CAD build for the part. Positions are in the model's coordinates, mm. Coordinates: 2 decimals unless noted, no trailing zeros. Loops run counter-clockwise (first coordinate to the right, second up) from the corner with the lowest first, then second, coordinate; pieces in that order, holes last. Notation, with made-up numbers: (54, 16.25) -> (59, 16.25) arc R25 cw to (59, 36.25) -> close; hole circle Ø9 at (28, 35.5). An arc over 180 degrees is marked (long way). Write each question's results on one line, items separated by ' | '.
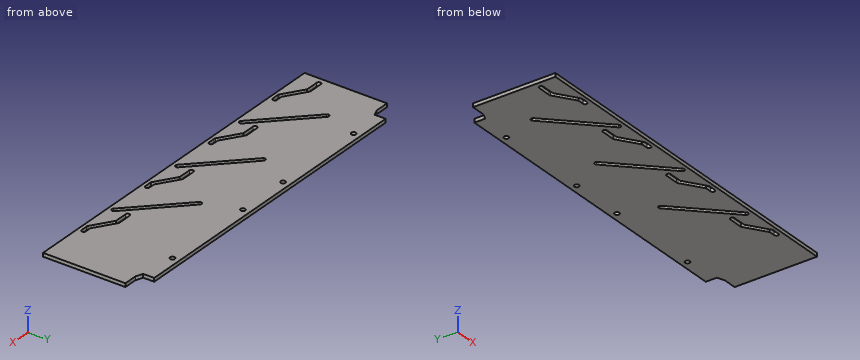
from build123d import *

# Parameters (mm, degrees)
SKETCH_1_W             = 260
SKETCH_1_H             = 70
EXTRUDE_1_DEPTH        = 2.6
SKETCH_2_R             = 1.7
CUT_EXTRUDE_1_DEPTH    = 135.654223848
SKETCH_3_R             = 1.3
CUT_EXTRUDE_2_DEPTH    = 135.654223848
CUT_EXTRUDE_4_DEPTH    = 135.654223848
PATTERN_LINEAR_2_COUNT = 3
PATTERN_LINEAR_2_PITCH = 63.333333333
CUT_EXTRUDE_3_DEPTH    = 135.654223848
PATTERN_LINEAR_1_COUNT = 4
PATTERN_LINEAR_1_PITCH = 63.333333333


with BuildPart() as part:
    # 草图1 → 凸台-拉伸1 (new body)
    with BuildSketch(Plane.XY):
        Rectangle(SKETCH_1_W, SKETCH_1_H)
    extrude(amount=EXTRUDE_1_DEPTH)

    # 草图2 → 切除-拉伸1 (cut, through all)
    with BuildSketch(Plane.XY.offset(2.6)):
        with Locations((-90, 30)):
            Circle(SKETCH_2_R)
        with Locations((-20, 30)):
            Circle(SKETCH_2_R)
        with Locations((20, 30)):
            Circle(SKETCH_2_R)
        with Locations((90, 30)):
            Circle(SKETCH_2_R)
        Polygon((-130, 25), (-130, 35), (-115, 35), (-115, 27), (-120, 25), align=None)
        Polygon((130, 25), (130, 35), (115, 35), (115, 27), (120, 25), align=None)
    extrude(amount=-CUT_EXTRUDE_1_DEPTH, mode=Mode.SUBTRACT)

    # 草图3 → 切除-拉伸2 (cut, through all)
    with BuildSketch(Plane.XY.offset(2.6)):
        with Locations((-61.666666667, -31)):
            Circle(SKETCH_3_R)
        with Locations((1.666666667, -31)):
            Circle(SKETCH_3_R)
        with Locations((65, -31)):
            Circle(SKETCH_3_R)
    extrude(amount=-CUT_EXTRUDE_2_DEPTH, mode=Mode.SUBTRACT)

    # 草图5 → 切除-拉伸4 (cut, through all)
    with BuildSketch(Plane.XY.offset(2.6)):
        with BuildLine():
            Line((-62.727326838, -32.060660172), (-98.727326838, 3.939339828))
            ThreePointArc((-98.727326838, 3.939339828), (-98.727326838, 6.060660172), (-96.606006495, 6.060660172))
            Line((-96.606006495, 6.060660172), (-60.606006495, -29.939339828))
            ThreePointArc((-60.606006495, -29.939339828), (-60.606006495, -32.060660172), (-62.727326838, -32.060660172))
        make_face()
    cut_extrude_4 = extrude(amount=-CUT_EXTRUDE_4_DEPTH, mode=Mode.SUBTRACT)

    # 阵列(线性)2: 切除-拉伸4 ×3
    with Locations(*[(i * PATTERN_LINEAR_2_PITCH, 0, 0) for i in range(1, PATTERN_LINEAR_2_COUNT)]):
        add(cut_extrude_4, mode=Mode.SUBTRACT)

    # 草图4 → 切除-拉伸3 (cut, through all)
    with BuildSketch(Plane.XY.offset(2.6)):
        with BuildLine():
            Line((-125, -19.5), (-115, -19.5))
            ThreePointArc((-115, -19.5), (-114.565323777, -19.56436196), (-114.167949706, -19.751924558))
            Line((-114.167949706, -19.751924558), (-99.545836543, -29.5))
            Line((-99.545836543, -29.5), (-95, -29.5))
            ThreePointArc((-95, -29.5), (-93.5, -31), (-95, -32.5))
            Line((-95, -32.5), (-100, -32.5))
            ThreePointArc((-100, -32.5), (-100.434676223, -32.43563804), (-100.832050294, -32.248075442))
            Line((-100.832050294, -32.248075442), (-115.454163457, -22.5))
            Line((-115.454163457, -22.5), (-125, -22.5))
            ThreePointArc((-125, -22.5), (-126.5, -21), (-125, -19.5))
        make_face()
    cut_extrude_3 = extrude(amount=-CUT_EXTRUDE_3_DEPTH, mode=Mode.SUBTRACT)

    # 阵列(线性)1: 切除-拉伸3 ×4
    with Locations(*[(i * PATTERN_LINEAR_1_PITCH, 0, 0) for i in range(1, PATTERN_LINEAR_1_COUNT)]):
        add(cut_extrude_3, mode=Mode.SUBTRACT)


solid = part.part
1) Slice it at C-C (y = -11). Write the cut outline in (x, z).
Outcome:
outline: (-130, 0) -> (-83.79, 0) -> (-83.79, 2.6) -> (-130, 2.6) -> close; (-79.55, 0) -> (-20.45, 0) -> (-20.45, 2.6) -> (-79.55, 2.6) -> close; (-16.21, 0) -> (42.88, 0) -> (42.88, 2.6) -> (-16.21, 2.6) -> close; (47.12, 0) -> (130, 0) -> (130, 2.6) -> (47.12, 2.6) -> close
2) Drill centre lines: L1, parallel to Y at x = 30, z = 1.3; L2, parallel to Y at x = 67.5, z = 1.55; L3, parallel to Y at x = -90, z = 0.6. Where is each one in solid material? Low to high. Write a range as from..to.
Outcome:
L1: y = -35..-32.5, -29.5..1.88, 6.12..35 | L2: y = -35..-22.5, -19.5..35 | L3: y = -35..-4.79, -0.55..28.3, 31.7..35
3) Pin check, flat tip, straight feed: pin 1 (1.3 mm diameter, centred on y = 32.5, z = 1.5, fed in from +X). Stop position of the tip, or through.
Outcome:
pin 1: stops at x = 115
4) Slice it at A-A (x = 70.5). Write the cut outline in (y, z).
Outcome:
outline: (-35, 0) -> (-22.5, 0) -> (-22.5, 2.6) -> (-35, 2.6) -> close; (-19.5, 0) -> (35, 0) -> (35, 2.6) -> (-19.5, 2.6) -> close
5) Slice it at B-B (z = 1.9). Count the separate pieces of the cut face and the enclosed holes in it, then the cut area to 3 significant figures.
Outcome:
separate pieces: 1 | enclosed holes: 11 | area: 17,000 mm^2
6) Slice it at D-D (x = -45.5). Write the cut outline in (y, z).
Outcome:
outline: (-35, 0) -> (-26.91, 0) -> (-26.91, 2.6) -> (-35, 2.6) -> close; (-23.31, 0) -> (35, 0) -> (35, 2.6) -> (-23.31, 2.6) -> close
